Input: part model. Units: mm. Frame: model coordinates. Face numbers are marked on the shaded views. A direction names the side the tool comes from. Coordinates: 2 decimals unless noted, no trailing zeros. Write each loop counter-clockwise with the first axis right and the second up, starting at its lowest first coordinate (ties: lowest second). Pieces come first, ordered by that corner, then holes. Notation, with made-up numbers: (23.25, 33.5) - (46.25, 33.5) arc R30 ccw to (46.25, 70.5) - close; hole circle Ø2 at (-28.75, 56). An arc over 180 degrees is marked (long way). One line per question, with ' | ' between items. Start each with the question number.
1) Section query B-B on y = -0.5. Return loops of the section in (x, z), and give its area (3 significant figures).
2) Draft query along Y for the marked faces 4, 5 and 6. Return one class per face: released by +Y, released by -Y, zero draft, split by the parting line, or undercut.
3) First-contact query: P1, Ø1, axis at x = -4.5, z = -4, coming from the +Y side; P2, Ø1.5, axis at x = -1.5, y = 0.5, coming from the -Z side; P3, Ø4, axis at y = 4.5, z = -5.5, coming from the +X side. Flat tips, straight axial feed; report the tip coordinate or a pass-through.
4) Section query D-D on x = 2. Return loops of the section in (y, z).
5) Reachability of the marked faces 1, 2 and 3 from +Z, -Z, +X, -X, +Y, -Y: full face, straight path, thin tool, end or side. Return the list, or none.
6) Line query: line 1 (Y direction, x = 1, z = -6); line 2 (X direction, y = 1, z = 0.5); line 3 (Y direction, x = 6.5, z = 1). Output: solid intervals per line, ascending.
7) Section query A-A on x = 0. Return loops of the section in (y, z), and give its area (3 significant figures).
8) Section query C-C on z = 1. Return loops of the section in (x, y), and give its area (3 significant figures).
```python
from build123d import *

# Parameters (mm, degrees)
SKETCH1_W                = 6
SKETCH1_H                = 1.2
SKETCH1_W_2              = 1.2
SKETCH1_H_2              = 4.3
REVOLVE1_ANGLE           = 180
REVOLVE2_START           = 4.3
REVOLVE2_DEPTH           = 2.7
CUT_EXTRUDE1_DEPTH       = 10
CUT_EXTRUDE2_DEPTH       = 10
SKETCH5_W                = 2
SKETCH5_H                = 2
BOSS_EXTRUDE1_DEPTH      = 1.2
SKETCH6_W                = 1.2
SKETCH6_H                = 3
BOSS_EXTRUDE2_DEPTH      = 1.5
CHAMFER1_SIZE            = 0.5
CHAMFER1_OF_MIRROR1_SIZE = 0.5


# Read off the part's stored shape, not the designer's step: Revolve2
with BuildPart() as part:
    # Sketch1 → Revolve1 (revolve)
    with BuildSketch(Plane.XY):
        with Locations((3, -0.6)):
            Rectangle(SKETCH1_W, SKETCH1_H)
        with Locations((6.6, -0.6)):
            Rectangle(SKETCH1_W_2, SKETCH1_H)
        with Locations((6.6, 2.15)):
            Rectangle(SKETCH1_W_2, SKETCH1_H_2)
    revolve(axis=Axis((0, -1.2, 0), (0, 1, 0)), revolution_arc=REVOLVE1_ANGLE)

    # Revolve2 outline → Revolve2 (add)
    with BuildSketch(Plane(origin=(0, 0, 0), x_dir=(1, 0, 0), z_dir=(0, 1, 0)).offset(REVOLVE2_START)):
        with BuildLine():
            ThreePointArc((3.7, 6.176568627), (0, 7.2), (-3.7, 6.176568627))
            Line((-3.7, 6.176568627), (-3.7, 4.723346271))
            ThreePointArc((-3.7, 4.723346271), (0, 6), (3.7, 4.723346271))
            Line((3.7, 4.723346271), (3.7, 6.176568627))
        make_face()
    extrude(amount=REVOLVE2_DEPTH)

    # Sketch3 → Cut-Extrude1 (cut)
    with BuildSketch(Plane.XY):
        Polygon((-3.25, 1.5), (-0.75, 1.5), (-0.75, 2.5), (0.75, 2.5), (0.75, 1.5), (3.25, 1.5), (3.25, 0), (-3.25, 0), align=None)
    extrude(amount=-CUT_EXTRUDE1_DEPTH, mode=Mode.SUBTRACT)

    # Sketch4 → Cut-Extrude2 (cut)
    with BuildSketch(Plane(origin=(0, 0, 0), x_dir=(1, 0, 0), z_dir=(0, 1, 0))):
        with BuildLine():
            Line((-1.2, 0.8), (-1.2, 2.529822128))
            ThreePointArc((-1.2, 2.529822128), (-2.366431913, 1.496662955), (-2.8, 0))
            Line((-2.8, 0), (2.8, 0))
            ThreePointArc((2.8, 0), (2.366431913, 1.496662955), (1.2, 2.529822128))
            Line((1.2, 2.529822128), (1.2, 0.8))
            Line((1.2, 0.8), (-1.2, 0.8))
        make_face()
    extrude(amount=-CUT_EXTRUDE2_DEPTH, mode=Mode.SUBTRACT)

    # Sketch5 → Boss-Extrude1 (add)
    with BuildSketch(Plane(origin=(0, 0, 0), x_dir=(1, 0, 0), z_dir=(0, 1, 0))):
        with Locations((-3.8, -1)):
            Rectangle(SKETCH5_W, SKETCH5_H)
        with Locations((3.8, -1)):
            Rectangle(SKETCH5_W, SKETCH5_H)
    extrude(amount=-BOSS_EXTRUDE1_DEPTH)

    # Sketch6 → Boss-Extrude2 (add)
    with BuildSketch(Plane(origin=(6, 0, 0), x_dir=(0, 0, -1), z_dir=(1, 0, 0))):
        with Locations((-0.6, 1.55)):
            Rectangle(SKETCH6_W, SKETCH6_H)
    boss_extrude2 = extrude(amount=BOSS_EXTRUDE2_DEPTH)

    # Chamfer1
    chamfer1_edges = [part.edges().sort_by_distance(p)[0] for p in [
        (7.5, 1.55, 1.2),
    ]]
    chamfer(chamfer1_edges, length=CHAMFER1_SIZE)

    # Mirror1: Boss-Extrude2 across plane
    add(boss_extrude2.mirror(Plane(origin=(0, 0, 0), x_dir=(0, 0, 1), z_dir=(1, 0, 0))))

    # Chamfer1 of Mirror1
    chamfer1_of_mirror1_edges = [part.edges().sort_by_distance(p)[0] for p in [
        (-7.5, 1.55, 1.2),
    ]]
    chamfer(chamfer1_of_mirror1_edges, length=CHAMFER1_OF_MIRROR1_SIZE)


solid = part.part
```
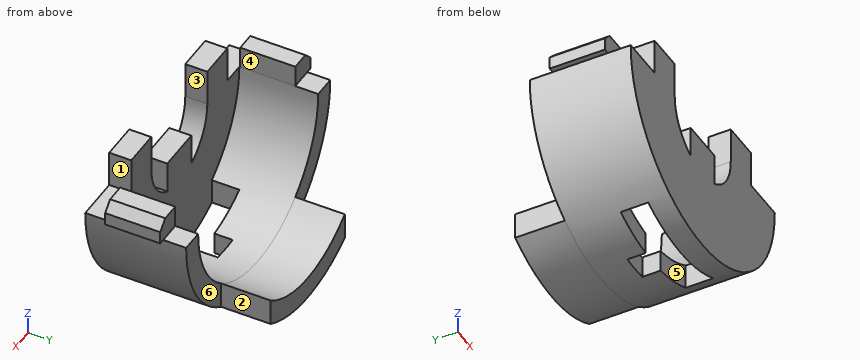
Answer key:
1) outline: (-7.2, 0) arc R7.2 ccw to (7.2, 0) - (4.8, 0) - (4.8, 2) - (2.8, 2) - (2.8, 0) arc R2.8 cw to (1.2, -2.53) - (1.2, -0.8) - (-1.2, -0.8) - (-1.2, -2.53) arc R2.8 cw to (-2.8, 0) - (-2.8, 2) - (-4.8, 2) - (-4.8, 0) - close | area: 81.7 mm²
2) face 4: zero draft | face 5: undercut | face 6: released by +Y
3) P1: y = 4.3 | P2: z = -7.14 | P3: x = 6.29
4) outline: (-1.2, -6.92) - (0, -6.92) - (0, -1.96) - (-1.2, -1.96) - close; (1.5, -6.92) - (7, -6.92) - (7, -5.66) - (1.5, -5.66) - close
5) face 1: +Z, +X, +Y, -Y | face 2: +Z, -Z, +X, +Y | face 3: +Z, +Y, -Y
6) line 1: -1.2 to 0, 1.5 to 7 | line 2: -7.5 to -6, 6 to 7.5 | line 3: 0.05 to 3.05
7) outline: (-1.2, -7.2) - (0, -7.2) - (0, -0.8) - (-1.2, -0.8) - close; (2.5, -7.2) - (7, -7.2) - (7, -6) - (2.5, -6) - close | area: 13.1 mm²
8) outline: (-7.2, 0.05) - (-6, 0.05) - (-6, 3.05) - (-7.2, 3.05) - close; (-4.8, -1.2) - (-2.8, -1.2) - (-2.8, 0) - (-4.8, 0) - close; (2.8, -1.2) - (4.8, -1.2) - (4.8, 0) - (2.8, 0) - close; (6, 0.05) - (7.2, 0.05) - (7.2, 3.05) - (6, 3.05) - close | area: 12.0 mm²
